from build123d import *

# Parameters (mm, degrees)
F0_R     = 19.05
F1_DEPTH = 76.2
F2_W     = 12.7
F2_H     = 69.85
F3_DEPTH = 38.1
F4_R     = 4.7625
F5_DEPTH = 12.7


with BuildPart() as f1:
    # F0 (on Top) → F1 (new body)
    with BuildSketch(Plane.XY):
        Circle(F0_R)
    extrude(amount=F1_DEPTH)

    # F2 (on Front) → F3 (join)
    with BuildSketch(Plane.XZ):
        with Locations((0, 41.275)):
            Rectangle(F2_W, F2_H)
    extrude(amount=F3_DEPTH)

    # F4 (on Right) → F5 (cut, symmetric)
    with BuildSketch(Plane.YZ):
        with Locations((-28.575, 63.5)):
            Circle(F4_R)
        with Locations((-28.575, 19.05)):
            Circle(F4_R)
    extrude(amount=F5_DEPTH, both=True, mode=Mode.SUBTRACT)


solid = f1.part
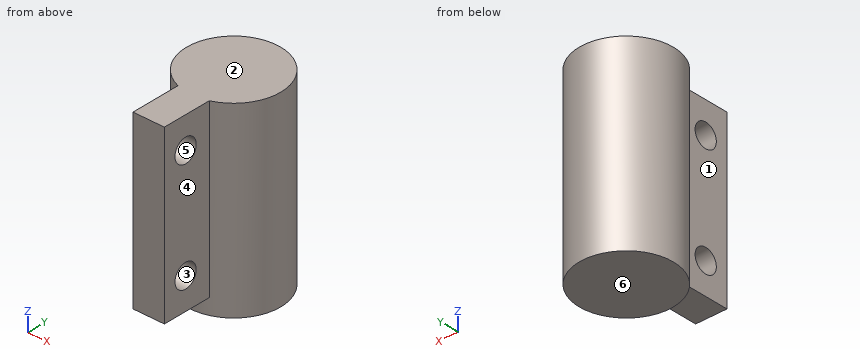
Work out the finished part from the listing and answer in its coordinate system (mm). Face numbers are marked on the shaded views. A direction names the side the tool comes from. Round coordinates to 2 decimals unless told otherwise and drop trailing zeros. Write each loop counter-clockwise with the first axis right and the second up, starting at its lowest first coordinate (ties: lowest second). Pieces come first, ordered by that corner, then holes. Notation, with made-up numbers: (10, 58.25) - (43, 58.25) arc R36 cw to (43, 92.25) - close; hole circle Ø3 at (35.5, 81). An arc over 180 degrees is marked (long way). Answer in a Markdown table with one row per item. Add a question column.
1. A cutting plane is placed at D-D, the plane z = 13. Determine the outline of the cut face in (x, y).
2. The mould has two halves that part along Z. Classify the marked faces 3, 4, 5 and 6: +Z half, -Z half, draft (parallel to the pull), parting line (faces both ways), or undercut.
3. A cutting plane is placed at B-B, the plane x = 0. Count the separate pieces of the cut face and the enclosed holes in it, and give its area (3 significant figures).
4. Given pin 1 (15 mm diameter, centred on y = -28.575, z = 19.05, fed in from -X); pin 2 (3 mm diameter, centred on y = -22.5, z = 40.5, fed in from -X); pin 3 (6 mm diameter, centred on x = -5.5, z = 63.5, fed in from +Y); pin 4 (5.5 mm diameter, centred on y = -28.575, z = 63.5, fed in from -X), each flat-ended and moving along its own axis, determine where each tip first touches the part or whether it passes through.
5. A cutting plane is placed at C-C, the plane y = -32. Determine the outline of the cut face in (x, z).
6. A cutting plane is placed at A-A, the plane z = 63.5. Determine the outline of the cut face in (x, y), and give its area (3 significant figures).
7. For the marked faces 1 and 2, determine the directions among +Z, -Z, +X, -X, +Y, -Y from which every point of the face is accessible in a straight line to the end or side of a thin tool.
8. Find the intervals of material crossed by line 1 along Z through (x, y) = (1, -29.5); line 2 along Z through (x, y) = (-1, -31); line 3 along Y through (x, z) = (4, 64), in increasing order. Write a range as from..to.
Worked out:
| question | item | result |
|---|---|---|
| 1 | outline | (-6.35, -38.1) - (6.35, -38.1) - (6.35, -17.96) arc R19.05 ccw (long way) to (-6.35, -17.96) - close |
| 2 | face 3 | undercut |
| 2 | face 4 | draft |
| 2 | face 5 | undercut |
| 2 | face 6 | -Z half |
| 3 | separate pieces | 1 |
| 3 | enclosed holes | 2 |
| 3 | area | 4,090 mm^2 |
| 4 | pin 1 | x = -6.35 |
| 4 | pin 2 | x = -6.35 |
| 4 | pin 3 | y = 18.89 |
| 4 | pin 4 | through |
| 5 | outline | (-6.35, 6.35) - (6.35, 6.35) - (6.35, 15.74) - (-6.35, 15.74) - close; (-6.35, 22.36) - (6.35, 22.36) - (6.35, 60.19) - (-6.35, 60.19) - close; (-6.35, 66.81) - (6.35, 66.81) - (6.35, 76.2) - (-6.35, 76.2) - close |
| 6 | outline | (-6.35, -38.1) - (6.35, -38.1) - (6.35, -33.34) - (-6.35, -33.34) - close; (-6.35, -23.81) - (6.35, -23.81) - (6.35, -17.96) arc R19.05 ccw (long way) to (-6.35, -17.96) - close |
| 6 | area | 1,270 mm^2 |
| 7 | face 1 | +Z, -Z, -X, -Y |
| 7 | face 2 | +Z, +X, -X, +Y, -Y |
| 8 | line 1 | 6.35..14.38, 23.72..58.83, 68.17..76.2 |
| 8 | line 2 | 6.35..14.95, 23.15..59.4, 67.6..76.2 |
| 8 | line 3 | -38.1..-33.31, -23.84..18.63 |
